from build123d import *

# Parameters (mm, degrees)
BOSS_EXTRUDE1_DEPTH = 10
BOSS_EXTRUDE2_DEPTH = 2


with BuildPart() as part:
    # Sketch1 → Boss-Extrude1 (new body)
    with BuildSketch(Plane.XY):
        with BuildLine():
            Line((-52.370168415, -5.10038319), (-57.370168415, -5.10038319))
            Line((-57.370168415, -5.10038319), (-57.370168415, -0.10038319))
            Line((-57.370168415, -0.10038319), (-52.370168415, -0.10038319))
            ThreePointArc((-52.370168415, -0.10038319), (-49.54174129, 1.071189685), (-48.370168415, 3.89961681))
            Line((-48.370168415, 3.89961681), (-48.370168415, 9.195191959))
            Line((-48.370168415, 9.195191959), (-25.403732634, 12.883646701))
            ThreePointArc((-25.403732634, 12.883646701), (-23.981138375, 13.054361886), (-22.549472845, 13.111387389))
            Line((-22.549472845, 13.111387389), (22.549472845, 13.111387389))
            ThreePointArc((22.549472845, 13.111387389), (23.981138375, 13.054361886), (25.403732634, 12.883646701))
            Line((25.403732634, 12.883646701), (48.370168415, 9.195191959))
            Line((48.370168415, 9.195191959), (48.370168415, 3.89961681))
            ThreePointArc((48.370168415, 3.89961681), (49.54174129, 1.071189685), (52.370168415, -0.10038319))
            Line((52.370168415, -0.10038319), (57.370168415, -0.10038319))
            Line((57.370168415, -0.10038319), (57.370168415, -5.10038319))
            Line((57.370168415, -5.10038319), (52.370168415, -5.10038319))
            ThreePointArc((52.370168415, -5.10038319), (49.54174129, -6.271956065), (48.370168415, -9.10038319))
            Line((48.370168415, -9.10038319), (48.370168415, -14.395958339))
            Line((48.370168415, -14.395958339), (25.403732634, -18.084413081))
            ThreePointArc((25.403732634, -18.084413081), (23.981138375, -18.255128266), (22.549472845, -18.312153769))
            Line((22.549472845, -18.312153769), (-22.549472845, -18.312153769))
            ThreePointArc((-22.549472845, -18.312153769), (-23.981138375, -18.255128266), (-25.403732634, -18.084413081))
            Line((-25.403732634, -18.084413081), (-48.370168415, -14.395958339))
            Line((-48.370168415, -14.395958339), (-48.370168415, -9.10038319))
            ThreePointArc((-48.370168415, -9.10038319), (-49.54174129, -6.271956065), (-52.370168415, -5.10038319))
        make_face()
    extrude(amount=BOSS_EXTRUDE1_DEPTH)

    # Sketch2 → Boss-Extrude2 (add)
    with BuildSketch(Plane.XY.offset(10)):
        with BuildLine():
            Line((-2, 11.111387389), (-2, -16.312153769))
            Line((-2, -16.312153769), (-22.549472845, -16.312153769))
            ThreePointArc((-22.549472845, -16.312153769), (-23.822064428, -16.261464433), (-25.086592657, -16.109717602))
            Line((-25.086592657, -16.109717602), (-45.370168415, -12.852135455))
            Line((-45.370168415, -12.852135455), (-45.370168415, 7.651369075))
            Line((-45.370168415, 7.651369075), (-25.086592657, 10.908951222))
            ThreePointArc((-25.086592657, 10.908951222), (-23.822064428, 11.060698053), (-22.549472845, 11.111387389))
            Line((-22.549472845, 11.111387389), (-2, 11.111387389))
        make_face()
        with BuildLine():
            Line((2, 11.111387389), (2, -16.312153769))
            Line((2, -16.312153769), (22.549472845, -16.312153769))
            ThreePointArc((22.549472845, -16.312153769), (23.822064428, -16.261464433), (25.086592657, -16.109717602))
            Line((25.086592657, -16.109717602), (45.370168415, -12.852135455))
            Line((45.370168415, -12.852135455), (45.370168415, 7.651369075))
            Line((45.370168415, 7.651369075), (25.086592657, 10.908951222))
            ThreePointArc((25.086592657, 10.908951222), (23.822064428, 11.060698053), (22.549472845, 11.111387389))
            Line((22.549472845, 11.111387389), (2, 11.111387389))
        make_face()
    extrude(amount=BOSS_EXTRUDE2_DEPTH)


solid = part.part
Model file for the job. Use its own axes, mm. A direction names the side the tool comes from. Give positions to 0.01 mm unless a question says otherwise; leave off trailing zeros. Order: outer loops, then holes, each group sorted by start corner. A loop starts at its lowest first (then second) coordinate and runs counter-clockwise, first axis right, second up. Notation, with made-up numbers: (64.25, 79.25) - (103.25, 79.25) arc R12 cw to (103.25, 102.25) - close; hole circle Ø8 at (22, 82). An arc over 180 degrees is marked (long way). Write item = value, one per line. Start each with the question number.
1. Cut at C-C, the plane y = 1.5. List the corners of the cut face in (x, z), and give its area (3 significant figures).
2. Cut at A-A, the plane x = -8. List the corners of the cut face in (y, z), and give its area (3 significant figures).
3. Drop flat-ended pins along their axis: P1, Ø5.5, axis at x = -53.5, z = 3.5, coming from the -Y side; P2, Ø6, axis at x = 44, z = 3.5, coming from the +Y side; P3, Ø5.5, axis at x = 55.5, z = 6, coming from the -Y side. Give the stop position or say it passes through.
4. Cut at D-D, the plane x = 28. List the corners of the cut face in (y, z), and give its area (3 significant figures).
5. Which spindle directions (+Z, -Z, +X, -X, +Y, -Y) get a long thin tool onto all of the face, cutting with end or side? Do faces 1 (the flat face through (-35.37, 9.257, 10.986)), 2 (the flat face through (55, -5.1, 5)), 3 (the flat face through (-55, -5.1, 5)), 4 (the cylindrical face through (23.804, -16.263, 10.986)), 5 (the flat face through (-35.1, -14.5, 11)). Say none if no direction does.
6. Cut at B-B, the plane z = 4. List the corners of the cut face in (x, y), and give its area (3 significant figures).
7. Probe line 1 along X through (y, z) = (-11.5, 3.75); line 2 along Z through (x, y) = (-39.5, 9.5); line 3 along Y through (x, z) = (-27, 11). List the from-to ranges inside material, lowest first.
Taken from the geometry:
q1.outline = (-49.17, 0) - (49.17, 0) - (49.17, 10) - (45.37, 10) - (45.37, 12) - (2, 12) - (2, 10) - (-2, 10) - (-2, 12) - (-45.37, 12) - (-45.37, 10) - (-49.17, 10) - close
q1.area = 1,160 mm²
q2.outline = (-18.31, 0) - (13.11, 0) - (13.11, 10) - (11.11, 10) - (11.11, 12) - (-16.31, 12) - (-16.31, 10) - (-18.31, 10) - close
q2.area = 369 mm²
q3.P1 = -5.44
q3.P2 = 10.38
q3.P3 = -5.1
q4.outline = (-17.67, 0) - (12.47, 0) - (12.47, 10) - (10.44, 10) - (10.44, 12) - (-15.64, 12) - (-15.64, 10) - (-17.67, 10) - close
q4.area = 354 mm²
q5.face_1 = +Z, -X, +Y
q5.face_2 = +Z, -Z, +X, -Y
q5.face_3 = +Z, -Z, -X, -Y
q5.face_4 = +Z, +X, -Y
q5.face_5 = +Z, -X, -Y
q6.outline = (-57.37, -5.1) - (-52.37, -5.1) arc R4 cw to (-48.37, -9.1) - (-48.37, -14.4) - (-25.4, -18.08) arc R18 ccw to (-22.55, -18.31) - (22.55, -18.31) arc R18 ccw to (25.4, -18.08) - (48.37, -14.4) - (48.37, -9.1) arc R4 cw to (52.37, -5.1) - (57.37, -5.1) - (57.37, -0.1) - (52.37, -0.1) arc R4 cw to (48.37, 3.9) - (48.37, 9.2) - (25.4, 12.88) arc R18 ccw to (22.55, 13.11) - (-22.55, 13.11) arc R18 ccw to (-25.4, 12.88) - (-48.37, 9.2) - (-48.37, 3.9) arc R4 cw to (-52.37, -0.1) - (-57.37, -0.1) - close
q6.area = 2,950 mm²
q7.line_1 = -48.37 to 48.37
q7.line_2 = 0 to 10
q7.line_3 = -15.8 to 10.6
